The listing builds one solid part. Answer for the finished solid, in the listing's coordinates (mm). Face numbers are marked on the shaded views. A direction names the side the tool comes from. Round coordinates to 2 decimals unless told otherwise and drop trailing zeros. Write each loop counter-clockwise with the first axis right and the second up, starting at its lowest first coordinate (ties: lowest second). Pieces come first, ordered by that corner, then holes. Notation, with made-up numbers: (39, 34) - (81, 34) arc R27 cw to (81, 65) - close; hole circle Ø5 at (-20.75, -32). An arc over 180 degrees is marked (long way). Return JSON: item names as keys, results as strings. Group by question number.
(1) Section D-D, the plane z = -28 is taken. Write down the section's boundary in (x, y), then the cut area to 3 significant figures.
(2) Section A-A, the plane x = 0 is taken. Write down the section's boundary in (y, z), then the cut area to 3 significant figures.
(3) Each of these flat-tipped pins is pushed along its axis until it touches: pin 1 (4 mm diameter, centred on x = 6, y = 92.5, fed in from -Z); pin 2 (3 mm diameter, centred on x = 8, y = 67.5, fed in from -Z); pin 3 (3.5 mm diameter, centred on x = -15.5, y = 112, fed in from +Z). Where does it stop, or does it pass through?
(4) Find the intervals of material crossed by line 1 along X through (y, z) = (110.75, -28); line 2 along Y through (x, z) = (-8, 1); line 3 along Z through (x, y) = (-2, 40), in increasing order. Write a range as [from, to].
(5) Section C-C, the plane y = 8 is taken. Write down the section's boundary in (x, z).
(6) Section B-B, the plane z = -42 is taken. Write down the section's boundary in (x, y), then the cut area to 3 significant figures.
(7) Which of the six approach directions +Z, -Z, +X, -X, +Y, -Y give full straight-line access (tool end or side, diameter ignored) to the marked faces 1 and 2?
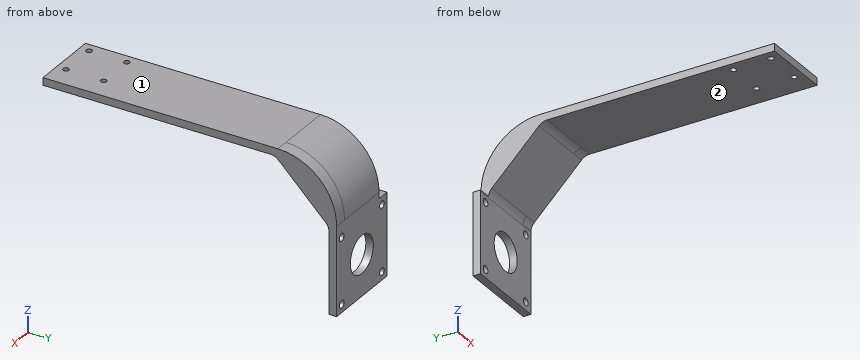
```python
from build123d import *

# Parameters (mm, degrees)
SKETCH1_W           = 24
SKETCH1_H           = 125
SKETCH1_R           = 1.25
BOSS_EXTRUDE1_DEPTH = 3.2
SKETCH2_W           = 24
SKETCH2_H           = 3.2
BOSS_EXTRUDE2_DEPTH = 42
SKETCH3_W           = 35
SKETCH3_H           = 35
SKETCH3_R           = 1.6
BOSS_EXTRUDE3_DEPTH = 3.2
SKETCH4_R           = 8
CUT_EXTRUDE1_DEPTH  = 3.2
CHAMFER1_SIZE       = 23
FILLET1_R           = 25
FILLET2_R           = 5
BOSS_EXTRUDE4_START = 5.5
BOSS_EXTRUDE4_DEPTH = 5.5


with BuildPart() as part:
    # Sketch1 → Boss-Extrude1 (new body)
    with BuildSketch(Plane.XY):
        with Locations((0, 50.5)):
            Rectangle(SKETCH1_W, SKETCH1_H)
        with Locations((-8, 8)):
            Circle(SKETCH1_R, mode=Mode.SUBTRACT)
        with Locations((8, 8)):
            Circle(SKETCH1_R, mode=Mode.SUBTRACT)
        with Locations((8, -8)):
            Circle(SKETCH1_R, mode=Mode.SUBTRACT)
        with Locations((-8, -8)):
            Circle(SKETCH1_R, mode=Mode.SUBTRACT)
    extrude(amount=BOSS_EXTRUDE1_DEPTH)

    # Sketch2 → Boss-Extrude2 (add)
    with BuildSketch(Plane(origin=(0, 0, 0), x_dir=(-1, 0, 0), z_dir=(0, 0, -1))):
        with Locations((0, 111.4)):
            Rectangle(SKETCH2_W, SKETCH2_H)
    extrude(amount=BOSS_EXTRUDE2_DEPTH)

    # Sketch3 → Boss-Extrude3 (add)
    with BuildSketch(Plane(origin=(0, 113, 0), x_dir=(1, 0, 0), z_dir=(0, 1, 0))):
        with Locations((0, 42)):
            Rectangle(SKETCH3_W, SKETCH3_H)
        with Locations(Location((14, 28, 0), (0, 0, 270))):
            Circle(SKETCH3_R, mode=Mode.SUBTRACT)
        with Locations(Location((14, 56, 0), (0, 0, 270))):
            Circle(SKETCH3_R, mode=Mode.SUBTRACT)
        with Locations(Location((-14, 56, 0), (0, 0, 270))):
            Circle(SKETCH3_R, mode=Mode.SUBTRACT)
        with Locations(Location((-14, 28, 0), (0, 0, 270))):
            Circle(SKETCH3_R, mode=Mode.SUBTRACT)
    extrude(amount=-BOSS_EXTRUDE3_DEPTH)

    # Sketch4 → Cut-Extrude1 (cut)
    with BuildSketch(Plane.XZ.offset(-109.8)):
        with Locations(Location((0, -42, 0), (0, 0, 270))):
            Circle(SKETCH4_R)
    extrude(amount=-CUT_EXTRUDE1_DEPTH, mode=Mode.SUBTRACT)

    # Chamfer1
    chamfer1_edges = [part.edges().sort_by_distance(p)[0] for p in [
        (0, 109.8, 0),
    ]]
    chamfer(chamfer1_edges, length=CHAMFER1_SIZE)

    # Fillet1
    fillet1_edges = [part.edges().sort_by_distance(p)[0] for p in [
        (0, 113, 3.2),
    ]]
    fillet(fillet1_edges, radius=FILLET1_R)

    # Fillet2
    fillet2_edges = [part.edges().sort_by_distance(p)[0] for p in [
        (0, 109.8, -23),
        (0, 86.8, 0),
    ]]
    fillet(fillet2_edges, radius=FILLET2_R)

    # Sketch7 → Boss-Extrude4 (add)
    with BuildSketch(Plane(origin=(12, 0, 0), x_dir=(0, 0, -1), z_dir=(1, 0, 0)).offset(BOSS_EXTRUDE4_START)):
        with BuildLine():
            Line((24.5, 113), (21.8, 113))
            ThreePointArc((21.8, 113), (4.12233047, 105.67766953), (-3.2, 88))
            Line((-3.2, 88), (-3.2, -12))
            Line((-3.2, -12), (0, -12))
            Line((0, -12), (0, 84.728932188))
            ThreePointArc((0, 84.728932188), (0.380602337, 86.64234935), (1.464466094, 88.264466094))
            Line((1.464466094, 88.264466094), (21.535533906, 108.335533906))
            ThreePointArc((21.535533906, 108.335533906), (22.896551906, 109.302386098), (24.5, 109.767281103))
            Line((24.5, 109.767281103), (24.5, 113))
        make_face()
    extrude(amount=-BOSS_EXTRUDE4_DEPTH)


solid = part.part
```
Working result:
{
 "1": {"outline": "(-17.5, 109.8) - (-15.6, 109.8) - (-15.6, 113) - (-17.5, 113) - close; (-12.4, 109.8) - (12.4, 109.8) - (12.4, 113) - (-12.4, 113) - close; (15.6, 109.8) - (17.5, 109.8) - (17.5, 113) - (15.6, 113) - close", "area": "91.5 mm^2"},
 "2": {"outline": "(-12, 0) - (84.73, 0) arc R5 cw to (88.26, -1.46) - (108.34, -21.54) arc R5 cw to (109.8, -25.07) - (109.8, -34) - (113, -34) - (113, -21.8) arc R25 ccw to (88, 3.2) - (-12, 3.2) - close; (109.8, -59.5) - (113, -59.5) - (113, -50) - (109.8, -50) - close", "area": "671 mm^2"},
 "3": {"pin 1": "stops at z = -7.7", "pin 2": "stops at z = 0", "pin 3": "stops at z = -24.5"},
 "4": {"line 1": "x = [-17.5, -15.6], [-12.4, 12.4], [15.6, 17.5]", "line 2": "y = [-12, -9.25], [-6.75, 6.75], [9.25, 98.25]", "line 3": "z = [0, 3.2]"},
 "5": {"outline": "(-12, 0) - (-9.25, 0) - (-9.25, 3.2) - (-12, 3.2) - close; (-6.75, 0) - (6.75, 0) - (6.75, 3.2) - (-6.75, 3.2) - close; (9.25, 0) - (17.5, 0) - (17.5, 3.2) - (9.25, 3.2) - close"},
 "6": {"outline": "(-17.5, 109.8) - (-8, 109.8) - (-8, 113) - (-17.5, 113) - close; (8, 109.8) - (17.5, 109.8) - (17.5, 113) - (8, 113) - close", "area": "60.8 mm^2"},
 "7": {"face 1": "+Z, +X, -X, +Y, -Y", "face 2": "-Z, +X, -X, -Y"}
}
